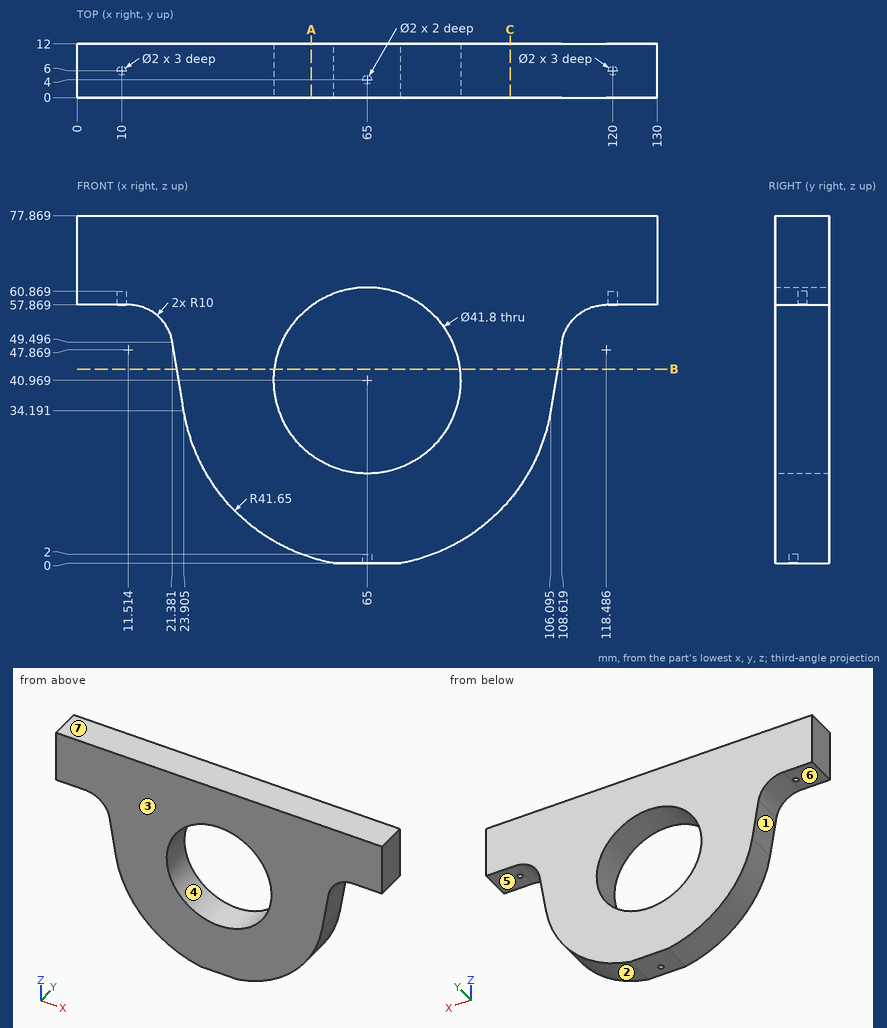
Study the drawing (mm; zero at the part's minimum x, y, z) and answer. A direction names the side the tool comes from. Give positions to 0.01 mm unless a question says otherwise; leave off trailing zeros. Write each loop counter-clockwise with the first axis right and the second up, starting at its lowest first coordinate (ties: lowest second). Pieces come first, ordered by that corner, then holes. Notation, with made-up numbers: (6, 18) -> (30, 18) arc R16 ccw to (30, 40) -> close; hole circle Ø6 at (65, -10.75). An arc over 180 degrees is marked (long way). Answer as a JSON object with one key per item and string values. Group by question number.
1) Find section B-B (z = 43.5). Write down the section's boundary in (x, y).
2) Find section C-C (x = 97). Write down the section's boundary in (y, z).
3) Find section A-A (x = 52.5). Write down the section's boundary in (y, z).
4) Each of these flat-tipped pins is pushed along its axis until it touches: P1, Ø5, axis at y = 5.5, z = 34, coming from the +X side (1 decimal); P2, Ø0.6, axis at x = 119.5, y = 6, coming from the -Z side; P3, Ø1, axis at y = 9.5, z = 19, coming from the -X side. Where does it stop, or does it pass through?
5) The mould has two halves that part along X. Classify the marked faces 1, 2, 3 and 4: +X half, -X half, draft (parallel to the pull), parting line (faces both ways), or undercut.
6) A tool of negligible diameter and unlimited length cuts with its end or side. For the marked faces 5, 6 and 7, from which of +Z, -Z, +X, -X, +Y, -Y can it reach the whole face along a straight path? Write none if from no direction.
7) Consider L1, parallel to X at y = 3.5, z = 55.5 (1 decimal); L2, parallel to X at y = 1.25, z = 22 (1 decimal); L3, parallel to Z at x = 120, y = 10. Determine where each line is inside the solid, lowest interval first. Write a range as from..to.
Values follow:
{
 "1": {"outline": "(22.37, 0) -> (44.25, 0) -> (44.25, 12) -> (22.37, 12) -> close; (85.75, 0) -> (107.63, 0) -> (107.63, 12) -> (85.75, 12) -> close"},
 "2": {"outline": "(0, 14.31) -> (12, 14.31) -> (12, 77.87) -> (0, 77.87) -> close"},
 "3": {"outline": "(0, 1.24) -> (12, 1.24) -> (12, 24.22) -> (0, 24.22) -> close; (0, 57.72) -> (12, 57.72) -> (12, 77.87) -> (0, 77.87) -> close"},
 "4": {"P1": "stops at x = 106.5", "P2": "stops at z = 60.87", "P3": "stops at x = 29.31"},
 "5": {"face 1": "-X half", "face 2": "+X half", "face 3": "draft", "face 4": "undercut"},
 "6": {"face 5": "-Z, +X, +Y, -Y", "face 6": "-Z, -X, +Y, -Y", "face 7": "+Z, +X, -X, +Y, -Y"},
 "7": {"L1": "x = 18..50, 80..112", "L2": "x = 27.9..56.2, 73.8..102.1", "L3": "z = 57.87..77.87"}
}
